```python
from build123d import *

# Parameters (mm, degrees)
SKETCH1_R           = 20.6375
BOSS_EXTRUDE1_DEPTH = 15.875
CHAMFER1_SIZE       = 1.27


with BuildPart() as part:
    # Sketch1 → Boss-Extrude1 (new body)
    with BuildSketch(Plane.XY):
        Polygon((0, 29.329393675), (-25.4, 14.664696837), (-25.4, -14.664696837), (0, -29.329393675), (25.4, -14.664696837), (25.4, 14.664696837), align=None)
        Circle(SKETCH1_R, mode=Mode.SUBTRACT)
    extrude(amount=BOSS_EXTRUDE1_DEPTH)

    # Chamfer1
    chamfer1_edges = [part.edges().sort_by_distance(p)[0] for p in [
        (-25.4, 0, 15.875),
        (-12.7, -21.997045256, 15.875),
        (12.7, -21.997045256, 15.875),
        (-20.6375, 0, 15.875),
        (25.4, 0, 15.875),
        (12.7, 21.997045256, 15.875),
        (-12.7, 21.997045256, 15.875),
    ]]
    chamfer(chamfer1_edges, length=CHAMFER1_SIZE)


solid = part.part
```
Model file for the job. Use its own axes, mm. Coordinates: 2 decimals unless noted, no trailing zeros. Write each loop counter-clockwise with the first axis right and the second up, starting at its lowest first coordinate (ties: lowest second). Pieces come first, ordered by that corner, then holes. Notation, with made-up numbers: (77, 71.25) - (105, 71.25) arc R9 cw to (105, 82.25) - close; hole circle Ø11 at (55.25, -2). An arc over 180 degrees is marked (long way). One line per item, written item: value. Start each with the question number.
1. Probe line 1 (Y direction, x = 0, z = 7); line 2 (Y direction, x = -11.5, z = 8.75); line 3 (X direction, y = -18, z = 3.5). List the from-to ranges inside material, lowest first. Write a range as from..to.
2. Mould opens along Y. For faces 1 (the flat face through (12.52, -22.1, 7.2)), 2 (the cylindrical face through (-4.474, -20.147, 7.2)), 3 (the flat face through (12.556, 21.337, 15.249)), 4 (the flat face through (-24.756, 0.205, 15.249)) say: released by +Y, released by -Y, zero draft, split by the parting line, or undercut.
3. Slice it at B-B (z = 8.5). Write the cut outline in (x, y) (1 decimal), plus the area to 3 significant figures.
4. Flat gauge pin, fed straight in: pin 1 (8 mm diameter, centred on x = 0, z = 7, fed in from -Y). Where does the tip first touch, or does it go through?
5. Slice it at A-A (y = 0). Write the cut outline in (x, z) (1 decimal).
Answers below:
1. line 1: y = -29.33..-20.64, 20.64..29.33
1. line 2: y = -22.69..-17.14, 17.14..22.69
1. line 3: x = -19.62..-10.09, 10.09..19.62
2. face 1: released by -Y
2. face 2: undercut
2. face 3: released by +Y
2. face 4: zero draft
3. outline: (-25.4, -14.7) - (0, -29.3) - (25.4, -14.7) - (25.4, 14.7) - (0, 29.3) - (-25.4, 14.7) - close; hole circle Ø41.3 at (0, 0)
3. area: 897 mm^2
4. pin 1: stops at y = -29.33
5. outline: (-25.4, 0) - (-20.6, 0) - (-20.6, 14.6) - (-21.9, 15.9) - (-24.1, 15.9) - (-25.4, 14.6) - close; (20.6, 0) - (25.4, 0) - (25.4, 14.6) - (24.1, 15.9) - (21.9, 15.9) - (20.6, 14.6) - close
